Part print with two shaded views. Sizes in mm from the minimum x, y, z corner. A direction names the side the tool comes from. Give positions to 0.01 mm unless a question says otherwise; leave off trailing zeros. Write each loop counter-clockwise with the first axis right and the second up, starting at its lowest first coordinate (ties: lowest second). Pieces come first, ordered by that corner, then holes. Notation, with made-up numbers: (0.5, 86.5) - (49.5, 86.5) arc R15 cw to (49.5, 102.5) - close; hole circle Ø3 at (88.25, 29). An arc over 180 degrees is marked (long way). Answer as a JSON object with one key per item and string values.
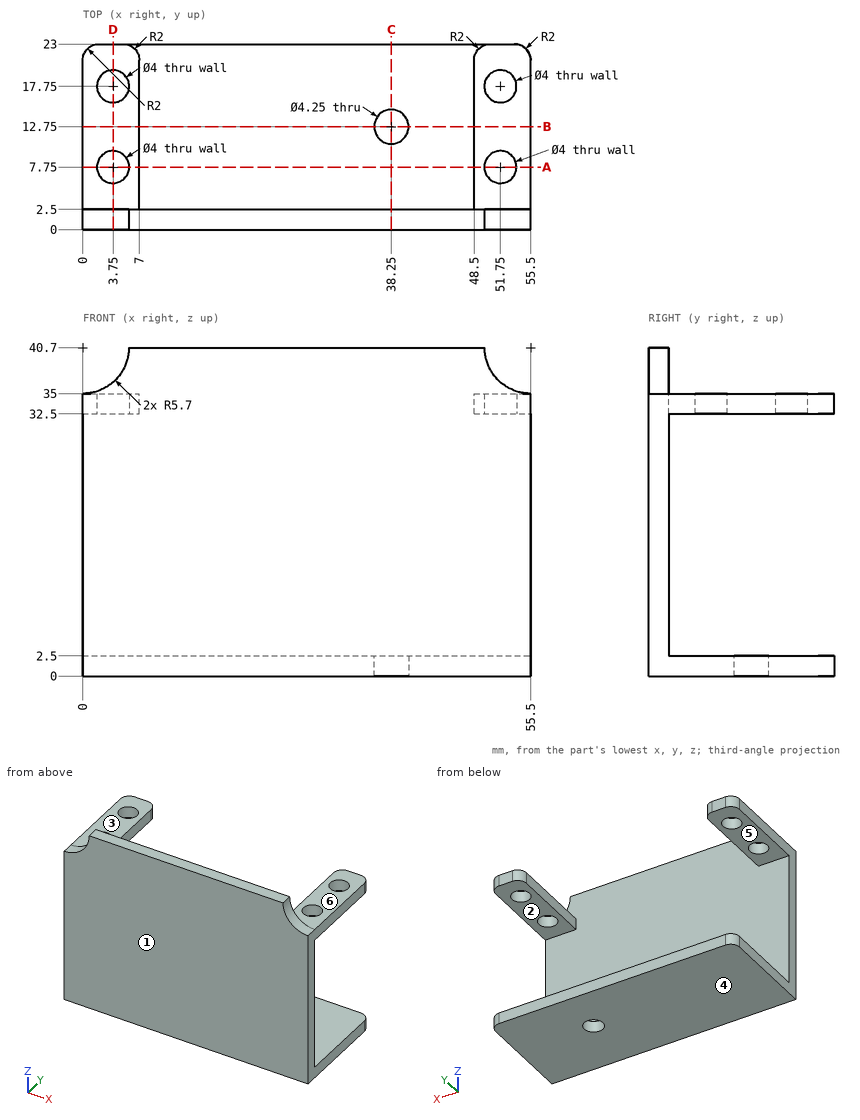
(1) Pull direction Z, two halves, no side cores. Call the marked faces 4, 5 and 6: pulls with the +Z half, pulls with the -Z half, needs draft (parallel to the pull), parting line crosses it, or undercut.
Answer key:
{"face 4": "pulls with the -Z half", "face 5": "undercut", "face 6": "pulls with the +Z half"}
(2) Saw through at B-B, the plane y = 12.75. Give the cut face in (x, z) (3 decimals).
Answer key:
{"outline": "(0, 0) - (36.125, 0) - (36.125, 2.5) - (0, 2.5) - close; (0, 32.5) - (7, 32.5) - (7, 35) - (0, 35) - close; (40.375, 0) - (55.5, 0) - (55.5, 2.5) - (40.375, 2.5) - close; (48.5, 32.5) - (55.5, 32.5) - (55.5, 35) - (48.5, 35) - close"}
(3) Saw through at D-D, the plane x = 3.75. Give the cut face in (y, z), and give its area (3 significant figures).
Answer key:
{"outline": "(0, 0) - (23, 0) - (23, 2.5) - (2.5, 2.5) - (2.5, 32.5) - (5.75, 32.5) - (5.75, 35) - (2.5, 35) - (2.5, 36.41) - (0, 36.41) - close; (9.75, 32.5) - (15.75, 32.5) - (15.75, 35) - (9.75, 35) - close; (19.75, 32.5) - (23, 32.5) - (23, 35) - (19.75, 35) - close", "area": "174 mm²"}
(4) Probe L1, parallel to Y at x = 3.75, z = 34.5; L2, parallel to Z at x = 4.5, y = 13.75; L3, parallel to Z at x = 4.5, y = 7. List the from-to ranges inside material, lowest first. Write a range as [from, to].
Answer key:
{"L1": "y = [0, 5.75], [9.75, 15.75], [19.75, 23]", "L2": "z = [0, 2.5], [32.5, 35]", "L3": "z = [0, 2.5]"}
(5) Saw through at C-C, the plane x = 38.25. Give the cut face in (y, z) (3 decimals), and give its area (3 significant figures).
Answer key:
{"outline": "(0, 0) - (10.625, 0) - (10.625, 2.5) - (2.5, 2.5) - (2.5, 40.7) - (0, 40.7) - close; (14.875, 0) - (23, 0) - (23, 2.5) - (14.875, 2.5) - close", "area": "142 mm²"}
(6) Flat gauge pins, fed straight in: P1, Ø11.5, axis at x = 30, z = 28.5, coming from the +Y side; P2, Ø5.5, axis at x = 2, y = 12.5, coming from the +Z side; P3, Ø2.5, axis at x = 3.75, y = 7.75, coming from the +Z side. Where does each tip first touch, or does it go through?
Answer key:
{"P1": "stops at y = 2.5", "P2": "stops at z = 35", "P3": "stops at z = 2.5"}
(7) Saw through at A-A, the plane y = 7.75. Give the cut face in (x, z), and give its area (3 significant figures).
Answer key:
{"outline": "(0, 0) - (55.5, 0) - (55.5, 2.5) - (0, 2.5) - close; (0, 32.5) - (1.75, 32.5) - (1.75, 35) - (0, 35) - close; (5.75, 32.5) - (7, 32.5) - (7, 35) - (5.75, 35) - close; (48.5, 32.5) - (49.75, 32.5) - (49.75, 35) - (48.5, 35) - close; (53.75, 32.5) - (55.5, 32.5) - (55.5, 35) - (53.75, 35) - close", "area": "154 mm²"}
(8) 3-axis set-ups, long thin cutter, end or side, ignore diameter. For the marked faces 1, 2 and 3: which of +Z, -Z, +X, -X, +Y, -Y reach the whole face in a straight line?
Answer key:
{"face 1": "+Z, -Z, +X, -X, -Y", "face 2": "+X, -X, +Y", "face 3": "+Z, +X, -X, +Y"}
